The listing builds one solid part. Answer for the finished solid, in the listing's coordinates (mm). A direction names the side the tool comes from. Coordinates: 2 decimals unless noted, no trailing zeros. Write each loop counter-clockwise with the first axis right and the second up, starting at its lowest first coordinate (ties: lowest second). Pieces come first, ordered by that corner, then holes. Notation, with made-up numbers: M 69,25 L 114,25 A14 cw 114,47 Z; hole C 19.5,73 d9. An arc over 180 degrees is marked long. Answer as CSV lines item,"result". Start each with the question number.
```python
from build123d import *

# Parameters (mm, degrees)
SKETCH_W     = 115
SKETCH_H     = 165
SKETCH_R     = 5
PAD_DEPTH    = 10
SKETCH001_W  = 10
SKETCH001_H  = 165
PAD001_DEPTH = 60
SKETCH002_W  = 10
SKETCH002_H  = 60
PAD002_DEPTH = 300


with BuildPart() as part:
    # Sketch (on Face1 of Copydouble_beam_01) → Pad (new body)
    with BuildSketch(Plane.XZ.offset(375)):
        with Locations((89.390244, 162.5)):
            Rectangle(SKETCH_W, SKETCH_H)
        with Locations((51.890244, 225)):
            Circle(SKETCH_R, mode=Mode.SUBTRACT)
        with Locations((126.890244, 100)):
            Circle(SKETCH_R, mode=Mode.SUBTRACT)
        with Locations((51.890244, 100)):
            Circle(SKETCH_R, mode=Mode.SUBTRACT)
        with Locations((126.890244, 225)):
            Circle(SKETCH_R, mode=Mode.SUBTRACT)
    extrude(amount=PAD_DEPTH)

    # Sketch001 (on Face10 of Pad) → Pad001 (join)
    with BuildSketch(Plane.XZ.offset(385)):
        with Locations((89.390244, 162.5)):
            Rectangle(SKETCH001_W, SKETCH001_H)
    extrude(amount=PAD001_DEPTH)

    # Sketch002 (on Face9 of Pad001) → Pad002 (join)
    with BuildSketch(Plane.XY.offset(245)):
        with Locations((89.390244, -415)):
            Rectangle(SKETCH002_W, SKETCH002_H)
    extrude(amount=PAD002_DEPTH)


solid = part.part
```
1) The part is cut by section C-C (z = 343.5). Determine the outline of the cut face in (x, y), then the cut area to 3 significant figures.
2) For a pull along X with two mould halves and no side action, classify faces 4 (the face through (120, -385, 164)), 5 (the face through (84.39, -415, 309)), 6 (the face through (131.66, -379.93, 101.5)) as +X half, -X half, draft (parallel to the pull), parting line (faces both ways), or undercut.
3) The part is cut by section B-B (x = 61). Determine the outline of the cut face in (y, z).
4) Which of the six approach directions +Z, -Z, +X, -X, +Y, -Y give full straight-line access (tool end or side, diameter ignored) to faces 1 (the face through (58, -385, 164)), 2 (the face through (94.39, -415, 309)), 3 (the face through (89, -385, 393))?
5) Each of these flat-tipped pins is pushed along its axis until it touches: P1, Ø16, axis at x = 132.5, z = 203.5, coming from the -Y side; P2, Ø10, axis at y = -391.5, z = 447.5, coming from the +X side; P3, Ø5, axis at x = 89.5, z = 378, coming from the +Y side. Where does it stop, or does it pass through?
6) Find the intervals of material crossed by line 1 (Z direction, x = 129, y = -381.5); line 2 (X direction, y = -410, z = 238.5); line 3 (Y direction, x = 91, z = 432.5), in increasing order. Write a range as from..to.
7) The part is cut by section A-A (z = 225). Determine the outline of the cut face in (x, y).
Completed:
1,outline,"M 84.39,-445 L 94.39,-445 L 94.39,-385 L 84.39,-385 Z"
1,area,"600 mm²"
2,face 4,"draft"
2,face 5,"-X half"
2,face 6,"undercut"
3,outline,"M -385,80 L -375,80 L -375,245 L -385,245 Z"
4,face 1,"+Z, -Z, -X, -Y"
4,face 2,"+Z, -Z, +X, -Y"
4,face 3,"+Z, +X, -X, +Y"
5,P1,"y = -385"
5,P2,"x = 94.39"
5,P3,"y = -385"
6,line 1,"80..95.47, 104.53..220.47, 229.53..245"
6,line 2,"84.39..94.39"
6,line 3,"-445..-385"
7,outline,"M 31.89,-385 L 46.89,-385 L 46.89,-375 L 31.89,-375 Z; M 56.89,-385 L 84.39,-385 L 84.39,-445 L 94.39,-445 L 94.39,-385 L 121.89,-385 L 121.89,-375 L 56.89,-375 Z; M 131.89,-385 L 146.89,-385 L 146.89,-375 L 131.89,-375 Z"
